Source: CAD feature listing. Evaluate the final solid. Frame: model axes, mm. Face numbers are marked on the shaded views. A direction names the side the tool comes from. Coordinates: 2 decimals unless noted, no trailing zeros. Order: outer loops, then holes, each group sorted by start corner. A loop starts at its lowest first (then second) coordinate and runs counter-clockwise, first axis right, second up.
```python
from build123d import *

# Parameters (mm, degrees)
SKETCH1_W                = 200
SKETCH1_H                = 60
BOSS_EXTRUDE1_DEPTH      = 25
SKETCH3_R                = 13.55
CUT_EXTRUDE1_DEPTH       = 7
CUT_EXTRUDE3_DEPTH       = 108.354552768
CUT_EXTRUDE7_DEPTH       = 45
FILLET8_R                = 5
SKETCH13_W               = 227.671202294
SKETCH13_H               = 68.392794906
SKETCH13_W_2             = 126
SKETCH13_H_2             = 41.42
CUT_EXTRUDE8_DEPTH       = 108.354552768
SKETCH14_W               = 12
SKETCH14_H               = 41.42
CUT_EXTRUDE9_DEPTH       = 131.573720174
CUT_EXTRUDE10_DEPTH      = 77.508930198
SKETCH19_W               = 126
SKETCH19_H               = 24.105748896
BOSS_EXTRUDE2_DEPTH      = 13
CUT_EXTRUDE11_DEPTH      = 77.508930198
CUT_EXTRUDE12_DEPTH      = 13
SKETCH22_W               = 58
SKETCH22_H               = 23.025801555
BOSS_EXTRUDE3_DEPTH      = 8
SKETCH24_W               = 40
SKETCH24_H               = 49.525748896
CUT_EXTRUDE13_DEPTH      = 4
CUT_EXTRUDE14_START      = -3
CUT_EXTRUDE14_DEPTH      = 3
CUT_EXTRUDE15_DEPTH      = 94.769991499
CUT_EXTRUDE15_DEPTH_BACK = 3
SKETCH27_R               = 2.05
CUT_EXTRUDE16_DEPTH      = 92.698728521


# Read off the part's stored shape, not the designer's step: Cut-Extrude14
with BuildPart() as part:
    # Sketch1 → Boss-Extrude1 (new body)
    with BuildSketch(Plane.XY):
        Rectangle(SKETCH1_W, SKETCH1_H)
    extrude(amount=BOSS_EXTRUDE1_DEPTH)

    # Sketch3 → Cut-Extrude1 (cut)
    with BuildSketch(Plane(origin=(0, 0, 0), x_dir=(-1, 0, 0), z_dir=(0, 0, -1))):
        with Locations((-45, 0)):
            Circle(SKETCH3_R)
        with Locations((45, 0)):
            Circle(SKETCH3_R)
    extrude(amount=-CUT_EXTRUDE1_DEPTH, mode=Mode.SUBTRACT)

    # Sketch6 → Cut-Extrude3 (cut, through all)
    with BuildSketch(Plane(origin=(0, 0, 0), x_dir=(-1, 0, 0), z_dir=(0, 0, -1))):
        Polygon((-100, 15.531551678), (-87.020750536, 30), (-100, 30), align=None)
        Polygon((-89.003501814, -30), (-100, -15.090940283), (-100, -30), align=None)
        Polygon((100, -30), (100, -15.090940283), (89.003501814, -30), align=None)
        Polygon((100, 30), (87.020750536, 30), (100, 15.531551678), align=None)
    extrude(amount=-CUT_EXTRUDE3_DEPTH, mode=Mode.SUBTRACT)

    # Sketch11 → Cut-Extrude7 (cut)
    with BuildSketch(Plane(origin=(0, 0, 0), x_dir=(-1, 0, 0), z_dir=(0, 0, -1))):
        Polygon((8.001444911, 30), (-99.028209758, 30), (-99.028209758, 24.58), (8.001444911, 24.58), (98.384596387, 24.58), (98.384596387, 30), align=None)
    extrude(amount=-CUT_EXTRUDE7_DEPTH, mode=Mode.SUBTRACT)

    # Fillet8
    fillet8_edges = [part.edges().sort_by_distance(p)[0] for p in [
        (100, 0.220305698, 25),
        (-100, 0.220305698, 25),
        (0, -30, 25),
        (-94.501750907, -22.545470141, 25),
        (94.501750907, -22.545470141, 25),
        (-95.941442184, 20.055775839, 25),
        (95.941442184, 20.055775839, 25),
        (0, 24.58, 25),
    ]]
    fillet(fillet8_edges, radius=FILLET8_R)

    # Sketch13 → Cut-Extrude8 (cut, through all)
    with BuildSketch(Plane(origin=(0, 0, 0), x_dir=(-1, 0, 0), z_dir=(0, 0, -1))):
        with Locations((1.665204381, -2.689234518)):
            Rectangle(SKETCH13_W, SKETCH13_H)
        with Locations((0, 2.71)):
            Rectangle(SKETCH13_W_2, SKETCH13_H_2, mode=Mode.SUBTRACT)
    extrude(amount=-CUT_EXTRUDE8_DEPTH, mode=Mode.SUBTRACT)

    # Sketch14 → Cut-Extrude9 (cut, through all)
    with BuildSketch(Plane(origin=(63, 0, 0), x_dir=(0, 0, -1), z_dir=(1, 0, 0))):
        with Locations((-19, 2.71)):
            Rectangle(SKETCH14_W, SKETCH14_H)
    extrude(amount=-CUT_EXTRUDE9_DEPTH, mode=Mode.SUBTRACT)

    # Sketch15 → Cut-Extrude10 (cut, through all)
    with BuildSketch(Plane(origin=(0, 23.42, 0), x_dir=(1, 0, 0), z_dir=(0, 1, 0))):
        Polygon((63, -6.5), (0, -13), (63, -13), align=None)
        Polygon((-63, -6.5), (0, -13), (-63, -13), align=None)
    extrude(amount=-CUT_EXTRUDE10_DEPTH, mode=Mode.SUBTRACT)

    # Sketch19 → Boss-Extrude2 (add)
    with BuildSketch(Plane(origin=(0, 0, 0), x_dir=(-1, 0, 0), z_dir=(0, 0, -1))):
        with Locations((0, -30.052874448)):
            Rectangle(SKETCH19_W, SKETCH19_H)
    extrude(amount=-BOSS_EXTRUDE2_DEPTH)

    # Sketch20 → Cut-Extrude11 (cut, through all)
    with BuildSketch(Plane(origin=(0, -18, 0), x_dir=(1, 0, 0), z_dir=(0, 1, 0))):
        Polygon((-63, -6.5), (-63, -13), (63, -13), (63, -6.5), (0, -13), align=None)
    extrude(amount=-CUT_EXTRUDE11_DEPTH, mode=Mode.SUBTRACT)

    # Sketch21 → Cut-Extrude12 (cut)
    with BuildSketch(Plane(origin=(0, 0, 0), x_dir=(-1, 0, 0), z_dir=(0, 0, -1))):
        Polygon((-63, -9.957970409), (-43, -42.105748896), (-63, -42.105748896), align=None)
        Polygon((-47.515984788, 23.42), (-63, 17.935984788), (-63, 23.42), align=None)
    cut_extrude12 = extrude(amount=-CUT_EXTRUDE12_DEPTH, mode=Mode.SUBTRACT)

    # Mirror1: Cut-Extrude12 across plane
    add(cut_extrude12.mirror(Plane(origin=(0, 0, 0), x_dir=(0, 0, 1), z_dir=(1, 0, 0))), mode=Mode.SUBTRACT)

    # Sketch22 → Boss-Extrude3 (add)
    with BuildSketch(Plane(origin=(0, 23.42, 0), x_dir=(1, 0, 0), z_dir=(0, 1, 0))):
        with Locations((0, 11.512900778)):
            Rectangle(SKETCH22_W, SKETCH22_H)
    boss_extrude3 = extrude(amount=-BOSS_EXTRUDE3_DEPTH)

    # Mirror2: Boss-Extrude3 across plane
    add(boss_extrude3.mirror(Plane(origin=(0, -9.342874448, 0), x_dir=(0, 0, 1), z_dir=(0, -1, 0))))

    # Sketch24 → Cut-Extrude13 (cut)
    with BuildSketch(Plane(origin=(0, 0, 0), x_dir=(-1, 0, 0), z_dir=(0, 0, -1))):
        with Locations((0, -9.342874448)):
            Rectangle(SKETCH24_W, SKETCH24_H)
    extrude(amount=-CUT_EXTRUDE13_DEPTH, mode=Mode.SUBTRACT)

    # Cut-Extrude14 outline → Cut-Extrude14 (cut)
    with BuildSketch(Plane(origin=(0, 23.42, 0), x_dir=(1, 0, 0), z_dir=(0, 1, 0)).offset(CUT_EXTRUDE14_START)):
        Polygon((29.370193256, -7.27376555), (29.370193256, 0), (29, 0), (29, 23.025801555), (-29, 23.025801555), (-29, 0), (-29.370193256, 0), (-29.370193256, -7.27376555), (0, -10.875770383), align=None)
    extrude(amount=CUT_EXTRUDE14_DEPTH, mode=Mode.SUBTRACT)

    # Sketch26 → Cut-Extrude15 (cut, two sides: drawn at the far end of the back side and taken through both)
    with BuildSketch(Plane.XZ.offset(42.105748896).offset(-CUT_EXTRUDE15_DEPTH_BACK)):
        Polygon((29, -230.630036101), (29, -23.025801555), (29, 0), (29.37, 0), (29.37, 7.84856116), (0, 10.878799255), (-29.37, 7.84856116), (-29.37, 0), (-29, 0), (-29, -23.025801555), (-29, -230.630036101), (-29, -645.838505193), (29, -645.838505193), align=None)
    extrude(amount=CUT_EXTRUDE15_DEPTH + CUT_EXTRUDE15_DEPTH_BACK, mode=Mode.SUBTRACT)

    # Sketch27 → Cut-Extrude16 (cut, through all)
    with BuildSketch(Plane(origin=(0, 20.42, 0), x_dir=(1, 0, 0), z_dir=(0, 1, 0))):
        with Locations(Location((17, -0.433798275, 0), (0, 0, 180))):
            Circle(SKETCH27_R)
        with Locations(Location((-17, -0.433798275, 0), (0, 0, 180))):
            Circle(SKETCH27_R)
        with Locations(Location((-17, 14.566201725, 0), (0, 0, 180))):
            Circle(SKETCH27_R)
        with Locations(Location((17, 14.566201725, 0), (0, 0, 180))):
            Circle(SKETCH27_R)
    extrude(amount=-CUT_EXTRUDE16_DEPTH, mode=Mode.SUBTRACT)


solid = part.part
```
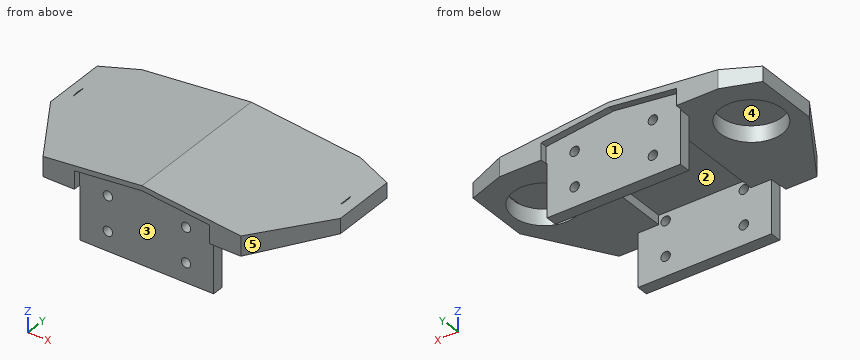
1. Section query A-A on z = -6. Return loops of the section in (x, y).
Findings:
outline: (-29, -39.11) - (29, -39.11) - (29, -34.11) - (-29, -34.11) - close; (-29, 15.42) - (29, 15.42) - (29, 20.42) - (-29, 20.42) - close
2. Draft query along Y for the marked faces 1, 2 and 3. Return one class per face: released by +Y, released by -Y, zero draft, split by the parting line, or undercut.
Findings:
face 1: released by +Y
face 2: undercut
face 3: released by -Y
3. Access query for the marked faces 4 and 5. Directions: +Z, -Z, +X, -X, +Y, -Y. A direction counts if a zero-diameter tool reaches every point of the face in a straight line with its end or side. Return the directions, or none.
Findings:
face 4: -Z
face 5: +Z, -Z, +X, -Y
4. Section query B-B on x = 17. Return loops of the section in (y, z).
Findings:
outline: (-42.11, 9.12) - (-39.11, 9.12) - (-39.11, 2.48) - (-34.11, 2.48) - (-34.11, 4) - (15.42, 4) - (15.42, 2.48) - (20.42, 2.48) - (20.42, 8.79) - (23.42, 8.79) - (23.42, 11.25) - (-42.11, 11.25) - close; (-39.11, -23.03) - (-34.11, -23.03) - (-34.11, -16.62) - (-39.11, -16.62) - close; (-39.11, -12.52) - (-34.11, -12.52) - (-34.11, -1.62) - (-39.11, -1.62) - close; (15.42, -23.03) - (20.42, -23.03) - (20.42, -16.62) - (15.42, -16.62) - close; (15.42, -12.52) - (20.42, -12.52) - (20.42, -1.62) - (15.42, -1.62) - close
5. Ray query, line 1 (Y direction, x = -27, z = -3); line 2 (Z direction, x = 17, y = -35.15); line 3 (Y direction, x = 45, z = 4). Return the intervals inside material, ascending.
Findings:
line 1: y = -39.11 to -34.11, 15.42 to 20.42
line 2: z = -23.03 to -16.62, -12.52 to -1.62, 2.48 to 11.25
line 3: y = -38.89 to -13.55, 13.55 to 23.42
6. Section query C-C on y = 0. Return loops of the section in (x, z).
Findings:
outline: (-63, 0) - (-58.55, 0) - (-58.55, 6.96) - (-63, 6.5) - close; (-58.15, 7) - (-31.45, 7) - (-31.45, 0) - (-20, 0) - (-20, 4) - (20, 4) - (20, 0) - (31.45, 0) - (31.45, 7) - (58.15, 7) - (0, 13) - close; (58.55, 0) - (63, 0) - (63, 6.5) - (58.55, 6.96) - close
7. Pin query (flat end, axial travel): P1, Ø6, axis at x = -35, y = 5, coming from the +Z side; P2, Ø5.5, axis at y = -36, z = -11, coming from the -X side; P3, Ø10, axis at x = 39, y = 2.5, coming from the +Z side; P4, Ø4, axis at y = -27, z = -3, coming from the -X side. Return the tip coordinate at first contact, or that it passes through.
Findings:
P1: stops at z = 9.7
P2: stops at x = -29
P3: stops at z = 9.49
P4: passes through
8. Section query D-D on x = -49.5. Return loops of the section in (y, z), plus the area to 3 significant figures.
Findings:
outline: (-31.66, 0) - (-12.78, 0) - (-12.78, 7) - (12.78, 7) - (12.78, 0) - (22.72, 0) - (22.72, 7.89) - (-31.66, 7.89) - close
area: 250 mm2
